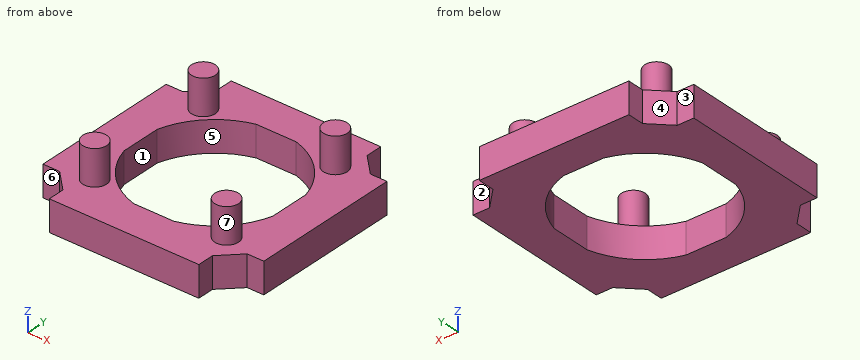
Autodesk Inventor part; units mm, degrees
ref_plane "Work Plane2" through (-40.9959, 0.8639, 22.2359) normal (0, 0, 1) x (1, 0, 0)
ref_plane "YZ Plane" through (0, 0, 0) normal (1, 0, 0) x (0, 1, 0)
ref_plane "XZ Plane" through (0, 0, 0) normal (0, 1, 0) x (-1, 0, 0)
ref_plane "Work Plane1" through (0, 0, 10) normal (0, 0, 1) x (1, 0, 0)
sketch "Sketch1" plane through (0, 0, 10) normal (0, 0, 1) x (1, 0, 0)
  line L0 (-4.0299, -0.3538) -> (-2.2322, 1.4439) construction
  arc A0 (-1.4439, 2.2322) -> (-2.2322, 1.4439) centre (-0.9299, 0.9299) ccw construction
  line L1 (-1.4439, 2.2322) -> (0.3538, 4.0299) construction
  line L2 (-37.8299, 42.8299) -> (-37.8299, 37.8299) construction
  line L3 (-37.8299, 37.8299) -> (-42.9208, 37.8299) construction
  line L4 (-37.8299, 42.2137) -> (-37.8299, 45.8299) construction
  line L5 (-37.8299, 45.8299) -> (-4.0299, 45.8299) construction
  line L6 (-4.0299, 45.8299) -> (-4.0299, 42.2137) construction
  line L7 (-4.0299, 4.0299) -> (0.3538, 4.0299)
  circle A1 centre (-20.9299, 20.9299) radius 17.5
  line L8 (-20.9299, 58.9723) -> (17.1124, 20.9299) construction
  line L9 (17.1124, 20.9299) -> (-20.9299, -17.1124) construction
  line L10 (-20.9299, -17.1124) -> (-58.9723, 20.9299) construction
  line L11 (-58.9723, 20.9299) -> (-20.9299, 58.9723) construction
  line L12 (-20.9299, 58.9723) -> (-20.9299, -17.1124) construction
  line L13 (17.1124, 20.9299) -> (-58.9723, 20.9299) construction
  line L14 (-20.9299, 58.9723) -> (32.8701, 58.9723) construction
  line L15 (-43.4299, 43.4299) -> (1.5701, 43.4299) construction
  line L16 (1.5701, 43.4299) -> (1.5701, -1.5701) construction
  line L17 (1.5701, -1.5701) -> (-43.4299, -1.5701) construction
  line L18 (-43.4299, -1.5701) -> (-43.4299, 43.4299) construction
  line L19 (-43.4299, 43.4299) -> (1.5701, -1.5701) construction
  line L20 (1.5701, 43.4299) -> (-43.4299, -1.5701) construction
  line L21 (-43.4299, 5.3876) -> (-43.4299, 36.4723)
  line L22 (-43.4299, 36.4723) -> (-36.4723, 43.4299)
  line L23 (-36.4723, 43.4299) -> (-5.3876, 43.4299)
  line L24 (-5.3876, 43.4299) -> (1.5701, 36.4723)
  line L25 (1.5701, 36.4723) -> (1.5701, 5.3876)
  line L26 (1.5701, 5.3876) -> (-5.3876, -1.5701)
  line L27 (-5.3876, -1.5701) -> (-36.4723, -1.5701)
  line L28 (-36.4723, -1.5701) -> (-43.4299, 5.3876)
  line L29 (-4.0299, 42.2137) -> (-37.8299, 42.2137)
  line L30 (-4.0299, -0.3538) -> (-4.0299, 4.0299)
  point P0 (-37.8299, 4.0299)
  point P1 (-20.9299, 20.9299)
  dimension "d18" = 53.8
  dimension "d19" = 45
  dimension "d20" = 53.8
  dimension "d21" = 45
  dimension "d22" = 45
extrude "Extrusion1" add sketch "Sketch1" along normal blind 7
sketch "Sketch2" plane through (0, 0, 17) normal (0, 0, 1) x (1, 0, 0)
  circle A0 centre (-35.9299, 35.9299) radius 3.0099 construction
  circle A1 centre (-5.93, 35.9299) radius 3.0099 construction
  circle A2 centre (-5.93, 5.93) radius 3.0099 construction
  circle A3 centre (-35.9299, 5.93) radius 3.0099 construction
  circle A4 centre (-35.9299, 35.9299) radius 2.7099
  circle A5 centre (-5.93, 35.9299) radius 2.7099
  circle A6 centre (-5.93, 5.93) radius 2.7099
  circle A7 centre (-35.9299, 5.93) radius 2.7099
  point P0 (0, 0)
  dimension "d_1" = 0.3
  dimension "d13" = 0.3
  dimension "d14" = 0.3
  dimension "d15" = 0.3
ref_plane "Work Plane2" through (-40.9959, 0.8639, 22.2359) normal (0, 0, 1) x (1, 0, 0)
extrude "Extrusion2" add sketch "Sketch2" along normal blind 8
sketch "Sketch3" plane through (0, 0, 10) normal (0, 0, -1) x (-1, 0, 0)
  line L0 (37.8299, -0.4701) -> (37.8299, 4.0299) construction
  line L1 (4.0299, 4.0299) -> (4.0299, -0.4701) construction
  line L2 (37.8299, -0.4701) -> (37.8299, 1.1886) construction
  line L3 (4.0299, -3.9701) -> (4.0299, -0.3538) construction
  line L4 (45.8299, 4.0299) -> (42.2137, 4.0299) construction
  line L5 (-0.3538, 4.0299) -> (-3.9701, 4.0299) construction
  line L6 (-3.9701, 37.8299) -> (-0.3538, 37.8299) construction
  line L7 (4.0299, 42.2137) -> (4.0299, 45.8299) construction
  line L8 (37.8299, 45.8299) -> (37.8299, 42.2137) construction
  line L9 (42.2137, 37.8299) -> (45.8299, 37.8299) construction
  line L10 (37.8299, 37.7299) -> (45.8299, 37.7299)
  line L11 (45.8299, 37.7299) -> (45.8299, 4.1299)
  line L12 (45.8299, 4.1299) -> (37.8299, 4.1299)
  line L13 (37.8299, 4.1299) -> (37.8299, 37.7299)
  line L14 (37.7299, 4.0299) -> (4.1299, 4.0299)
  line L15 (4.1299, 4.0299) -> (4.1299, -3.9701)
  line L16 (4.1299, -3.9701) -> (37.7299, -3.9701)
  line L17 (37.7299, -3.9701) -> (37.7299, 4.0299)
  line L18 (4.0299, 4.1299) -> (-3.9701, 4.1299)
  line L19 (-3.9701, 4.1299) -> (-3.9701, 37.7299)
  line L20 (-3.9701, 37.7299) -> (4.0299, 37.7299)
  line L21 (4.0299, 37.7299) -> (4.0299, 4.1299)
  line L22 (4.1299, 37.8299) -> (37.7299, 37.8299)
  line L23 (37.7299, 37.8299) -> (37.7299, 45.8299)
  line L24 (37.7299, 45.8299) -> (4.1299, 45.8299)
  line L25 (4.1299, 45.8299) -> (4.1299, 37.8299)
  point P0 (0, 0)
  dimension "d23" = 0.1
  dimension "d24" = 0.1
  dimension "d25" = 0.1
  dimension "d26" = 0.1
  dimension "d27" = 0.1
extrude "Extrusion3" add sketch "Sketch3" against normal up to surface (7 mm away)
sketch "Sketch4" plane through (0, 0, 17) normal (0, 0, 1) x (1, 0, 0)
  arc A0 (-16.3868, 4.0299) -> (-4.0299, 16.3868) centre (-20.9299, 20.9299) ccw
  line L0 (-25.4731, 4.0299) -> (-16.3868, 4.0299)
  arc A1 (-37.8299, 16.3868) -> (-25.4731, 4.0299) centre (-20.9299, 20.9299) ccw
  line L1 (-37.8299, 25.4731) -> (-37.8299, 16.3868)
  arc A2 (-25.4731, 37.8299) -> (-37.8299, 25.4731) centre (-20.9299, 20.9299) ccw
  line L2 (-16.3868, 37.8299) -> (-25.4731, 37.8299)
  arc A3 (-4.0299, 25.4731) -> (-16.3868, 37.8299) centre (-20.9299, 20.9299) ccw
  line L3 (-4.0299, 16.3868) -> (-4.0299, 25.4731)
  circle A4 centre (-5.93, 5.93) radius 2.7099
  circle A5 centre (-5.93, 35.9299) radius 2.7099
  circle A6 centre (-35.9299, 35.9299) radius 2.7099
  circle A7 centre (-35.9299, 5.93) radius 2.7099
  line L4 (3.9701, 4.1299) -> (0.3124, 4.1299)
  line L5 (3.9701, 37.7299) -> (3.9701, 4.1299)
  line L6 (0.3124, 37.7299) -> (3.9701, 37.7299)
  line L7 (0.3124, 37.7299) -> (-4.1299, 42.1723)
  line L8 (-4.1299, 45.8299) -> (-4.1299, 42.1723)
  line L9 (-37.7299, 45.8299) -> (-4.1299, 45.8299)
  line L10 (-37.7299, 42.1723) -> (-37.7299, 45.8299)
  line L11 (-37.7299, 42.1723) -> (-42.1723, 37.7299)
  line L12 (-45.8299, 37.7299) -> (-42.1723, 37.7299)
  line L13 (-45.8299, 4.1299) -> (-45.8299, 37.7299)
  line L14 (-42.1723, 4.1299) -> (-45.8299, 4.1299)
  line L15 (-42.1723, 4.1299) -> (-37.7299, -0.3124)
  line L16 (-37.7299, -3.9701) -> (-37.7299, -0.3124)
  line L17 (-4.1299, -3.9701) -> (-37.7299, -3.9701)
  line L18 (-4.1299, -0.3124) -> (-4.1299, -3.9701)
  line L19 (-4.1299, -0.3124) -> (0.3124, 4.1299)
  line L20 (-3.9299, 46.0299) -> (-3.9299, 42.2551)
  line L21 (-3.9299, 42.2551) -> (0.3953, 37.9299)
  line L22 (0.3953, 37.9299) -> (4.1701, 37.9299)
  line L23 (4.1701, 37.9299) -> (4.1701, 3.9299)
  line L24 (4.1701, 3.9299) -> (0.3953, 3.9299)
  line L25 (0.3953, 3.9299) -> (-3.9299, -0.3953)
  line L26 (-3.9299, -0.3953) -> (-3.9299, -4.1701)
  line L27 (-3.9299, -4.1701) -> (-37.9299, -4.1701)
  line L28 (-37.9299, -4.1701) -> (-37.9299, -0.3953)
  line L29 (-37.9299, -0.3953) -> (-42.2551, 3.9299)
  line L30 (-42.2551, 3.9299) -> (-46.0299, 3.9299)
  line L31 (-46.0299, 3.9299) -> (-46.0299, 37.9299)
  line L32 (-46.0299, 37.9299) -> (-42.2551, 37.9299)
  line L33 (-42.2551, 37.9299) -> (-37.9299, 42.2551)
  line L34 (-37.9299, 42.2551) -> (-37.9299, 46.0299)
  line L35 (-37.9299, 46.0299) -> (-3.9299, 46.0299)
  point P0 (0, 0)
  dimension "d30" = 0.2
extrude "Extrusion4" add sketch "Sketch4" against normal up to surface (7 mm away) contours L20 L21 L22 L23 L24 L25 L26 L27 L28 L29 L30 L31 L32 L33 L34 L35
equation "\"d13\" = d_1"
equation "\"d14\" = d_1"
equation "\"d15\" = d_1"
properties part number "50_Cube_Insert_Thorlabs"
Design review of the part built by this model. Coordinates are the model's own, in mm. Face numbers are marked on the shaded views. A direction names the side the tool comes from. Coordinates: 2 decimals unless noted, no trailing zeros. Order: outer loops, then holes, each group sorted by start corner. A loop starts at its lowest first (then second) coordinate and runs counter-clockwise, first axis right, second up. Notation, with made-up numbers: (73, -33.5) -> (98, -33.5) arc R21 cw to (98, -18.5) -> close; hole circle Ø5 at (-32, 62.5). An arc over 180 degrees is marked (long way). One line per item, written item: value.
1) Clearance check with flat-ended pins moving along their axes: P1, Ø3, axis at y = 44, z = 12, coming from the +X side; P2, Ø1.9, axis at x = -44, z = 12, coming from the -Y side; P3, Ø10, axis at x = -12, y = 20, coming from the +Z side; P4, Ø1.9, axis at x = 2.5, z = 12.5, coming from the +Y side. State where each tip first meets the part, or that it passes through.
Output values:
P1: stops at x = -3.93
P2: stops at y = 3.93
P3: passes through
P4: stops at y = 37.93
2) We need section D-D, the plane x = -8. Give the boundary of the cut face in (y, z).
Output values:
outline: (-4.17, 10) -> (9.14, 10) -> (9.14, 17) -> (7.68, 17) -> (7.68, 25) -> (4.18, 25) -> (4.18, 17) -> (-4.17, 17) -> close; (32.72, 10) -> (46.03, 10) -> (46.03, 17) -> (37.68, 17) -> (37.68, 25) -> (34.18, 25) -> (34.18, 17) -> (32.72, 17) -> close
3) Draft analysis for pull direction X (two halves, no side actions). For the marked faces 4, 5, 6 and 7, state which applies: +X half, -X half, draft (parallel to the pull), parting line (faces both ways), or undercut.
Output values:
face 4: -X half
face 5: undercut
face 6: draft
face 7: undercut
4) We need section C-C, the plane z = 11.5. Give the boundary of the cut face in (x, y), then the cut area to 3 significant figures.
Output values:
outline: (-46.03, 3.93) -> (-42.26, 3.93) -> (-37.93, -0.4) -> (-37.93, -4.17) -> (-3.93, -4.17) -> (-3.93, -0.4) -> (0.4, 3.93) -> (4.17, 3.93) -> (4.17, 37.93) -> (0.4, 37.93) -> (-3.93, 42.26) -> (-3.93, 46.03) -> (-37.93, 46.03) -> (-37.93, 42.26) -> (-42.26, 37.93) -> (-46.03, 37.93) -> close; hole (-37.83, 16.39) arc R17.5 ccw to (-25.47, 4.03) -> (-16.39, 4.03) arc R17.5 ccw to (-4.03, 16.39) -> (-4.03, 25.47) arc R17.5 ccw to (-16.39, 37.83) -> (-25.47, 37.83) arc R17.5 ccw to (-37.83, 25.47) -> close
area: 1,350 mm2
5) We need section A-A, the plane y = 23. Give the boundary of the cut face in (x, z), then the cut area to 3 significant figures.
Output values:
outline: (-46.03, 10) -> (-37.83, 10) -> (-37.83, 17) -> (-46.03, 17) -> close; (-4.03, 10) -> (4.17, 10) -> (4.17, 17) -> (-4.03, 17) -> close
area: 115 mm2
6) To check wall thickness, follow probe 1 along X at (y, z) = (18.5, 14.5); probe 2 along Y at (x, z) = (-22.5, 14.25); probe 3 along Z at (x, y) = (-6.5, 2.5). State the ranges of each line that lie inside material, in increasing order. Write a range as [from, to].
Output values:
probe 1: x = [-46.03, -37.83], [-4.03, 4.17]
probe 2: y = [-4.17, 4.03], [37.83, 46.03]
probe 3: z = [10, 17]
7) Machinability: for the marked faces 1, 2 and 3, which of the approach directions +Z, -Z, +X, -X, +Y, -Y give a long, thin tool a straight path to every point of the face, cutting with its end or side? Answer none if there is none.
Output values:
face 1: +Z, -Z
face 2: +Z, -Z, +X, +Y
face 3: +Z, -Z, -X, +Y
8) We need section B-B, the plane x = -24. Give the boundary of the cut face in (y, z), then the cut area to 3 significant figures.
Output values:
outline: (-4.17, 10) -> (4.03, 10) -> (4.03, 17) -> (-4.17, 17) -> close; (37.83, 10) -> (46.03, 10) -> (46.03, 17) -> (37.83, 17) -> close
area: 115 mm2
